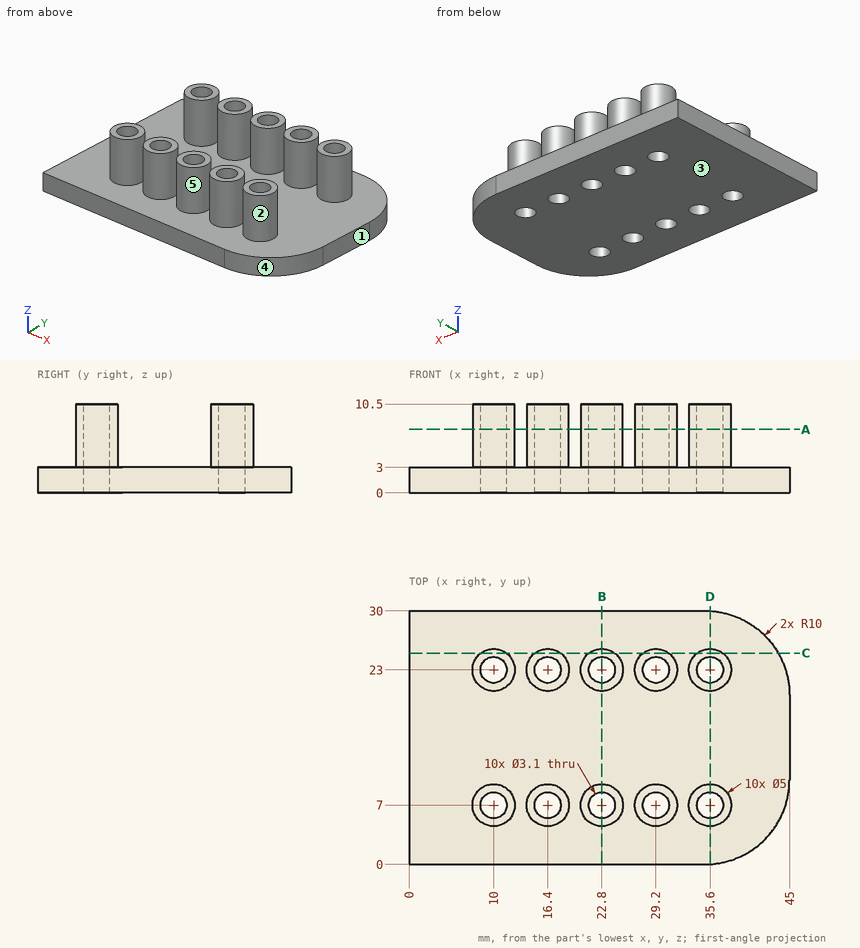
Verification items for this drawing (mm, ordinates from the low corner). A direction names the side the tool comes from. Round coordinates to 2 decimals unless told otherwise and drop trailing zeros. Order: outer loops, then holes, each group sorted by start corner. A loop starts at its lowest first (then second) coordinate and runs counter-clockwise, first axis right, second up. Notation, with made-up numbers: M 64.5,37 L 86.5,37 A22 cw 86.5,66 Z; hole C -16.5,-19.5 d5. An arc over 180 degrees is marked long. Answer in a Markdown table with one row per item. Add a question column.
Item 1: Sectioned sample at C-C, the plane y = 25. Enter the section's corners in (x, z).
Item 2: Draft check along Y on the marked faces 3, 4 and 5. Enter one of: released by +Y, released by -Y, zero draft, split by the parting line, or undercut.
Item 3: Material ranges on L1, parallel to Y at x = 10, z = 4.75; L2, parallel to Y at x = 21.5, z = 2.5; L3, parallel to X at y = 25, z = 6, recorded low to high. Write a range as [from, to].
Item 4: Depth check by flat-ended pin: pin 1 Ø2.5 at (x, y) = (22.8, 23) entering from -Z; pin 2 Ø5 at (y, z) = (5.5, 2.5) entering from +X; pin 3 Ø4 at (x, z) = (11, 7) entering from +Y; pin 4 Ø2 at (y, z) = (5, 8) entering from -X. Enter the tip coordinate at first touch or a pass-through.
Item 5: Set-up check for the marked faces 1 and 2: record each of +Z, -Z, +X, -X, +Y, -Y from which the full face is reachable in a straight line by a thin tool's end or side.
Item 6: Sectioned sample at B-B, the plane x = 22.8. Enter the section's corners in (y, z), plus the area to 3 significant figures.
Item 7: Sectioned sample at D-D, the plane x = 35.6. Enter the section's corners in (y, z).
Item 8: Sectioned sample at A-A, the plane z = 7.5. State how many separate pieces and enclosed holes the cut face has, plus the area to 3 significant figures.
Filled in:
| question | item | result |
|---|---|---|
| 1 | outline | M 0,0 L 43.66,0 L 43.66,3 L 37.1,3 L 37.1,10.5 L 34.1,10.5 L 34.1,3 L 30.7,3 L 30.7,10.5 L 27.7,10.5 L 27.7,3 L 24.3,3 L 24.3,10.5 L 21.3,10.5 L 21.3,3 L 17.9,3 L 17.9,10.5 L 14.9,10.5 L 14.9,3 L 11.5,3 L 11.5,10.5 L 8.5,10.5 L 8.5,3 L 0,3 Z |
| 2 | face 3 | zero draft |
| 2 | face 4 | released by -Y |
| 2 | face 5 | undercut |
| 3 | L1 | y = [4.5, 5.45], [8.55, 9.5], [20.5, 21.45], [24.55, 25.5] |
| 3 | L2 | y = [0, 6.16], [7.84, 22.16], [23.84, 30] |
| 3 | L3 | x = [8.5, 11.5], [14.9, 17.9], [21.3, 24.3], [27.7, 30.7], [34.1, 37.1] |
| 4 | pin 1 | passes through |
| 4 | pin 2 | stops at x = 44.8 |
| 4 | pin 3 | stops at y = 25.5 |
| 4 | pin 4 | stops at x = 7.71 |
| 5 | face 1 | +Z, -Z, +X, +Y, -Y |
| 5 | face 2 | +Z |
| 6 | outline | M 0,0 L 5.45,0 L 5.45,10.5 L 4.5,10.5 L 4.5,3 L 0,3 Z; M 8.55,0 L 21.45,0 L 21.45,10.5 L 20.5,10.5 L 20.5,3 L 9.5,3 L 9.5,10.5 L 8.55,10.5 Z; M 24.55,0 L 30,0 L 30,3 L 25.5,3 L 25.5,10.5 L 24.55,10.5 Z |
| 6 | area | 99.9 mm² |
| 7 | outline | M 0.02,0 L 5.45,0 L 5.45,10.5 L 4.5,10.5 L 4.5,3 L 0.02,3 Z; M 8.55,0 L 21.45,0 L 21.45,10.5 L 20.5,10.5 L 20.5,3 L 9.5,3 L 9.5,10.5 L 8.55,10.5 Z; M 24.55,0 L 29.98,0 L 29.98,3 L 25.5,3 L 25.5,10.5 L 24.55,10.5 Z |
| 8 | separate pieces | 10 |
| 8 | enclosed holes | 10 |
| 8 | area | 121 mm² |
